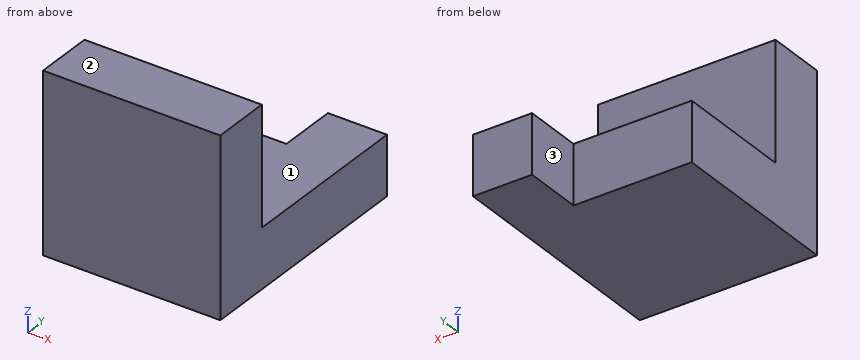
from build123d import *

# Parameters (mm, degrees)
ESBO_O1_W                = 60
ESBO_O1_H                = 20
RESSALTO_EXTRUS_O1_DEPTH = 40
ESBO_O2_W                = 60
ESBO_O2_H                = 60.417785093
RESSALTO_EXTRUS_O2_DEPTH = 20
ESBO_O3_W                = 20
ESBO_O3_H                = 20
RESSALTO_EXTRUS_O3_DEPTH = 20


with BuildPart() as part:
    # Esboço1 → Ressalto-extrusão1 (new body)
    with BuildSketch(Plane.XY):
        with Locations((30, 10)):
            Rectangle(ESBO_O1_W, ESBO_O1_H)
    extrude(amount=RESSALTO_EXTRUS_O1_DEPTH)

    # Esboço2 → Ressalto-extrusão2 (add)
    with BuildSketch(Plane(origin=(0, 0, 0), x_dir=(-1, 0, 0), z_dir=(0, 0, -1))):
        with Locations((-30, 30.208892547)):
            Rectangle(ESBO_O2_W, ESBO_O2_H)
    extrude(amount=RESSALTO_EXTRUS_O2_DEPTH)

    # Esboço3 → Ressalto-extrusão3 (add)
    with BuildSketch(Plane(origin=(0, 60.417785093, 0), x_dir=(1, 0, 0), z_dir=(0, 1, 0))):
        with Locations((50, 10)):
            Rectangle(ESBO_O3_W, ESBO_O3_H)
    extrude(amount=RESSALTO_EXTRUS_O3_DEPTH)


solid = part.part
Check sheet for the modelled part. Datum: model origin and axes. Units: mm. Face numbers are marked on the shaded views. A direction names the side the tool comes from. Give positions to 0.01 mm unless a question says otherwise; leave off trailing zeros. Order: outer loops, then holes, each group sorted by start corner. A loop starts at its lowest first (then second) coordinate and runs counter-clockwise, first axis right, second up. Notation, with made-up numbers: M -33.5,-12.5 L 6.5,-12.5 A19 ccw 6.5,-1.5 Z; hole C -35,87 d10. An arc over 180 degrees is marked long. Answer as CSV lines item,"result". Start each with the question number.
Item 1: Cross-section at C-C on y = 56. Enter the section's corners in (x, z).
Item 2: Cross-section at A-A on x = 46.5. Enter the section's corners in (y, z).
Item 3: Cross-section at B-B on z = -8. Enter the section's corners in (x, y).
Item 4: Cross-section at D-D on z = 23.5. Enter the section's corners in (x, y), plus the area to 3 significant figures.
Item 5: Thickness scan on line 1 (Z direction, x = 51.5, y = 39); line 2 (Y direction, x = 31.5, z = -9.5); line 3 (Y direction, x = 43, z = 18). Record the ranges inside material, lowest first. Write a range as [from, to].
Item 6: Gauge pin test, flat ends, axial feed: P1, Ø6, axis at x = 18, z = 2.5, coming from the +Y side; P2, Ø12, axis at y = 52, z = 9.5, coming from the -X side; P3, Ø10, axis at y = 67, z = -7, coming from the -X side; P4, Ø12, axis at x = 19.5, z = 20.5, coming from the +Y side. Record the tip position at first contact, or that the pin passes through.
Item 7: Tool access check on the marked faces 1, 2 and 3. Record the directions out of +Z, -Z, +X, -X, +Y, -Y that give a thin tool (end or side, any length) a straight path to the whole face; none if there is none.
Established:
1,outline,"M 0,-20 L 60,-20 L 60,0 L 0,0 Z"
2,outline,"M 0,-20 L 80.42,-20 L 80.42,0 L 20,0 L 20,40 L 0,40 Z"
3,outline,"M 0,0 L 60,0 L 60,80.42 L 40,80.42 L 40,60.42 L 0,60.42 Z"
4,outline,"M 0,0 L 60,0 L 60,20 L 0,20 Z"
4,area,"1,200 mm^2"
5,line 1,"z = [-20, 0]"
5,line 2,"y = [0, 60.42]"
5,line 3,"y = [0, 20]"
6,P1,"stops at y = 60.42"
6,P2,"passes through"
6,P3,"stops at x = 40"
6,P4,"stops at y = 20"
7,face 1,"+Z, +X, -X, +Y"
7,face 2,"+Z, +X, -X, +Y, -Y"
7,face 3,"+Z, -Z, -X, +Y"
